```python
from build123d import *

# Parameters (mm, degrees)
SKETCH1_R           = 3.175
BOSS_EXTRUDE1_DEPTH = 50.8
FILLET1_R           = 1.27
SKETCH4_R           = 2.38125
FILLET2_R           = 1.27


with BuildPart() as part:
    # Sketch1 → Boss-Extrude1 (new body)
    with BuildSketch(Plane(origin=(0, 0, 0), x_dir=(1, 0, 0), z_dir=(0, 1, 0))):
        with Locations(Location((0, 0, 0), (0, 0, 270))):
            Circle(SKETCH1_R)
    extrude(amount=BOSS_EXTRUDE1_DEPTH)

    # Fillet1
    fillet1_edges = [part.edges().sort_by_distance(p)[0] for p in [
        (0, 0, -3.175),
    ]]
    fillet(fillet1_edges, radius=FILLET1_R)

    # Sweep1: sweep along a path in Sketch2
    with BuildLine(Plane.XY) as sweep1_path:
        Line((0, 50.8), (0, 55.095962307))
    # Sketch4 → Sweep1 (sweep)
    with BuildSketch(Plane(origin=(0, 50.8, 0), x_dir=(1, 0, 0), z_dir=(0, 1, 0))):
        Circle(SKETCH4_R)
    sweep(path=sweep1_path.line)

    # Fillet2
    # the kernel refuses this fillet: 1.27 mm, written as the material it adds along each edge
    with BuildSketch(Plane(origin=(0, 50.8, 0), x_dir=(1, 0, 0), z_dir=(0, 0, 1))) as fillet2_piece_1:
        with BuildLine():
            CenterArc((3.65125, 1.17732151), FILLET2_R, 180, 67.975687163)
            Line((2.38125, 1.17732151), (2.35585, 1.17732151))
            Line((2.35585, 1.17732151), (2.35585, 0))
            Line((2.35585, 0), (2.38125, -0.0254))
            ThreePointArc((2.38125, -0.0254), (2.778125, -0.0254), (3.165475, -0.02354643))
            Line((3.165475, -0.02354643), (3.175, 0))
        make_face()
    revolve(axis=Axis((0, 50.8, 0), (0, 1, 0)))


solid = part.part
```
Verification items for the finished model (mm, model axes). A direction names the side the tool comes from. Round coordinates to 2 decimals unless told otherwise and drop trailing zeros. Write each loop counter-clockwise with the first axis right and the second up, starting at its lowest first coordinate (ties: lowest second). Pieces come first, ordered by that corner, then holes.
1. Section check B-B on x = 0. Enter the section's corners in (y, z) (3 decimals).
2. Access from +Z, -Z, +X, -X, +Y, -Y to the whole of each face (thin tool, end or side, straight path). Record for faces 1 (the cylindrical face through (-1.93, 25.69, -2.52)), 2 (the cylindrical face through (-1.89, 53.56, 1.45)).
3. Scan lines: L1, parallel to X at y = 29, z = -0.25; L2, parallel to Y at x = 2, z = 0.5; L3, parallel to Z at x = 0.5, y = 35.5. Record each from-to range of solid material in increasing order.
4. Gauge pin test, flat ends, axial feed: P1, Ø3, axis at y = 42.5, z = 1, coming from the +X side (3 decimals); P2, Ø1.5, axis at x = 1.5, y = 28.5, coming from the -Z side; P3, Ø2, axis at y = 24, z = 1.5, coming from the -X side. Record the tip position at first contact, or that the pin passes through.
5. Section check A-A on z = 0. Enter the section's corners in (x, y) (3 decimals), plus the area to 3 significant figures.
6. Section check C-C on y = 36.5. Enter the section's corners in (x, z) (3 decimals).
Answer:
1. outline: (0, -1.905) arc R1.27 ccw to (1.27, -3.175) - (50.8, -3.175) arc R1.27 cw to (51.977, -2.381) - (55.096, -2.381) - (55.096, 2.381) - (51.977, 2.381) arc R1.27 cw to (50.8, 3.175) - (1.27, 3.175) arc R1.27 ccw to (0, 1.905) - close
2. face 1: +Y, -Y
2. face 2: +Y
3. L1: x = -3.17 to 3.17
3. L2: y = 0.01 to 55.1
3. L3: z = -3.14 to 3.14
4. P1: stops at x = 3.175
4. P2: stops at z = -3.09
4. P3: stops at x = -3.14
5. outline: (-3.175, 1.27) arc R1.27 ccw to (-1.905, 0) - (1.905, 0) arc R1.27 ccw to (3.175, 1.27) - (3.175, 50.8) arc R1.27 cw to (2.381, 51.977) - (2.381, 55.096) - (-2.381, 55.096) - (-2.381, 51.977) arc R1.27 cw to (-3.175, 50.8) - close
5. area: 343 mm2
6. outline: circle Ø6.35 at (0, 0)
